Build history of the part. All positions in model axes, mm. A direction names the side the tool comes from. Coordinates: 2 decimals unless noted, no trailing zeros. Write each loop counter-clockwise with the first axis right and the second up, starting at its lowest first coordinate (ties: lowest second). Pieces come first, ordered by that corner, then holes.
```python
from build123d import *

# Parameters (mm, degrees)
SKETCH1_W           = 60
SKETCH1_H           = 80
BOSS_EXTRUDE4_DEPTH = 6
BOSS_EXTRUDE5_DEPTH = 25
SKETCH1_15_R        = 2
CUT_EXTRUDE1_DEPTH  = 25
SKETCH1_16_R        = 4
SKETCH1_16_R_2      = 2
CUT_EXTRUDE2_DEPTH  = 25
SKETCH1_18_R        = 4
SKETCH1_18_R_2      = 2
BOSS_EXTRUDE7_DEPTH = 3
FILLET1_R           = 10


with BuildPart() as part:
    # Sketch1 → Boss-Extrude4 (new body)
    with BuildSketch(Plane.XY):
        with Locations((30, 40)):
            Rectangle(SKETCH1_W, SKETCH1_H)
    extrude(amount=BOSS_EXTRUDE4_DEPTH)

    # Sketch1<12> → Boss-Extrude5 (add)
    with BuildSketch(Plane.XY):
        Polygon((5, 5), (5, 80), (0, 80), (0, 0), (60, 0), (60, 5), align=None)
    extrude(amount=BOSS_EXTRUDE5_DEPTH)

    # Sketch1<15> → Cut-Extrude1 (cut)
    with BuildSketch(Plane.XY):
        with Locations((50, 60)):
            Circle(SKETCH1_15_R)
        with Locations((15, 60)):
            Circle(SKETCH1_15_R)
    extrude(amount=CUT_EXTRUDE1_DEPTH, mode=Mode.SUBTRACT)

    # Sketch1<16> → Cut-Extrude2 (cut)
    # profile 1 of 2: a face of its own
    with BuildSketch(Plane.XY):
        with Locations((50, 60)):
            Circle(SKETCH1_16_R)
        with Locations((50, 60)):
            Circle(SKETCH1_16_R_2, mode=Mode.SUBTRACT)
    # profile 2 of 2: a face of its own
    with BuildSketch(Plane.XY):
        with Locations((15, 60)):
            Circle(SKETCH1_16_R)
        with Locations((15, 60)):
            Circle(SKETCH1_16_R_2, mode=Mode.SUBTRACT)
    extrude(amount=CUT_EXTRUDE2_DEPTH, mode=Mode.SUBTRACT)

    # Sketch1<18> → Boss-Extrude7 (add)
    # profile 1 of 2: a face of its own
    with BuildSketch(Plane.XY):
        with Locations((50, 60)):
            Circle(SKETCH1_18_R)
        with Locations((50, 60)):
            Circle(SKETCH1_18_R_2, mode=Mode.SUBTRACT)
    # profile 2 of 2: a face of its own
    with BuildSketch(Plane.XY):
        with Locations((15, 60)):
            Circle(SKETCH1_18_R)
        with Locations((15, 60)):
            Circle(SKETCH1_18_R_2, mode=Mode.SUBTRACT)
    extrude(amount=BOSS_EXTRUDE7_DEPTH)

    # Fillet1
    fillet1_edges = [part.edges().sort_by_distance(p)[0] for p in [
        (60, 0, 12.5),
        (0, 80, 12.5),
        (0, 0, 12.5),
    ]]
    fillet(fillet1_edges, radius=FILLET1_R)


solid = part.part
```
1. Probe line 1 along X through (y, z) = (60, 4.85); line 2 along Y through (x, z) = (15, 2.2); line 3 along Y through (x, z) = (45.5, 15). List the from-to ranges inside material, lowest first.
Computed values:
line 1: x = 0 to 11, 19 to 46, 54 to 60
line 2: y = 0 to 58, 62 to 80
line 3: y = 0 to 5
2. Saw through at C-C on z = 5. List the corners of the cut face in (x, y).
Computed values:
outline: (0, 10) arc R10 ccw to (10, 0) - (50, 0) arc R10 ccw to (60, 10) - (60, 80) - (10, 80) arc R10 ccw to (0, 70) - close; hole circle Ø8 at (15, 60); hole circle Ø8 at (50, 60)
3. Saw through at A-A on y = 60. List the corners of the cut face in (x, z), plus the area to 3 significant figures.
Computed values:
outline: (0, 0) - (13, 0) - (13, 3) - (11, 3) - (11, 6) - (5, 6) - (5, 25) - (0, 25) - close; (17, 0) - (48, 0) - (48, 3) - (46, 3) - (46, 6) - (19, 6) - (19, 3) - (17, 3) - close; (52, 0) - (60, 0) - (60, 6) - (54, 6) - (54, 3) - (52, 3) - close
area: 383 mm2
4. 3-axis set-ups, long thin cutter, end or side, ignore diameter. For faces 4 (the face through (49.133, 56.095, 4.479)), 5 (the face through (32, 43, 6)), 6 (the face through (30, 0, 12)): which of +Z, -Z, +X, -X, +Y, -Y reach the whole face in a straight line?
Computed values:
face 4: +Z
face 5: +Z, +X, +Y
face 6: +Z, -Z, +X, -X, -Y
5. Mould opens along Y. For faces 1 (the face through (2.85, 3.01, 12.68)), 2 (the face through (5, 41, 15)), 3 (the face through (14.133, 56.095, 4.479)) say: +Y half, -Y half, draft (parallel to the pull), parting line (faces both ways), or undercut.
Computed values:
face 1: -Y half
face 2: draft
face 3: undercut
6. Saw through at D-D on x = 26.5. List the corners of the cut face in (y, z).
Computed values:
outline: (0, 0) - (80, 0) - (80, 6) - (5, 6) - (5, 25) - (0, 25) - close
7. Saw through at B-B on x = 15. List the corners of the cut face in (y, z).
Computed values:
outline: (0, 0) - (58, 0) - (58, 3) - (56, 3) - (56, 6) - (5, 6) - (5, 25) - (0, 25) - close; (62, 0) - (80, 0) - (80, 6) - (64, 6) - (64, 3) - (62, 3) - close
8. Flat gauge pins, fed straight in: pin 1 (5 mm diameter, centred on y = 9, z = 11, fed in from -X); pin 2 (1 mm diameter, centred on x = 43.5, y = 33.5, fed in from +Z); pin 3 (15 mm diameter, centred on y = 28.5, z = 20, fed in from +X); pin 4 (5 mm diameter, centred on x = 50, y = 60, fed in from +Z). Where does each tip first touch, or does it go through?
Computed values:
pin 1: stops at x = 0
pin 2: stops at z = 6
pin 3: stops at x = 5
pin 4: stops at z = 3
